```python
from build123d import *

# Parameters (mm, degrees)
F0_R     = 8.5
F1_DEPTH = 4
F2_R     = 5
F3_DEPTH = 100
F4_W     = 4
F4_H     = 5
F8_R     = 1.5
F9_DEPTH = 109.1


with BuildPart() as f1:
    # F0 (on Top) → F1 (new body)
    with BuildSketch(Plane.XY):
        Circle(F0_R)
    extrude(amount=F1_DEPTH)

    # F2 (on Top) → F3 (join)
    with BuildSketch(Plane.XY):
        Circle(F2_R)
    extrude(amount=F3_DEPTH)

    # F4 (on Right) → F5 (revolve)
    with BuildSketch(Plane.YZ):
        with Locations((2, 102.5)):
            Rectangle(F4_W, F4_H)
    revolve(axis=Axis((0, 0, 102.5), (0, 0, -1)))

    # F6 (on Right) → F7 (revolve)
    with BuildSketch(Plane.YZ):
        with BuildLine():
            ThreePointArc((3, 105), (2.12132, 107.12132), (0, 108))
            Line((0, 108), (0, 105))
            Line((0, 105), (3, 105))
        make_face()
    revolve(axis=Axis((0, 0, 106.5), (0, 0, -1)))

    # F8 (on Top) → F9 (cut)
    with BuildSketch(Plane.XY):
        Circle(F8_R)
    extrude(amount=F9_DEPTH, mode=Mode.SUBTRACT)


solid = f1.part
```
Read the model definition and answer for the solid it produces. Units are mm, in the model's axes. A direction names the side the tool comes from. Coordinates: 2 decimals unless noted, no trailing zeros. Loops run counter-clockwise (first coordinate to the right, second up) from the corner with the lowest first, then second, coordinate; pieces in that order, holes last. Notation, with made-up numbers: (70, 69.25) - (82, 69.25) arc R12 ccw to (82, 89.25) - close; hole circle Ø3 at (34.5, 53). An arc over 180 degrees is marked (long way). Answer in a Markdown table with one row per item.
1. Find section C-C, the plane x = 6. Write down the section's boundary in (y, z), then the cut area to 3 significant figures.
Conclusion:
| item | result |
|---|---|
| outline | (-6.02, 0) - (6.02, 0) - (6.02, 4) - (-6.02, 4) - close |
| area | 48.2 mm² |
2. Straight lines are drawn through the part: line 1 (Y direction, x = 0, z = 45.5); line 2 (X direction, y = 4, z = 94.5). For each, find the intervals that lie inside material, in ascending order.
Conclusion:
| item | result |
|---|---|
| line 1 | y = -5 to -1.5, 1.5 to 5 |
| line 2 | x = -3 to 3 |
3. Given pin 1 (1.5 mm diameter, centred on x = -4.5, z = 54, fed in from +Y); pin 2 (5 mm diameter, centred on x = 1, z = 90, fed in from +Y); pin 3 (2 mm diameter, centred on y = -1.5, z = 89.5, fed in from -X), each flat-ended and moving along its own axis, determine where each tip first touches the part or whether it passes through.
Conclusion:
| item | result |
|---|---|
| pin 1 | stops at y = 3.31 |
| pin 2 | stops at y = 5 |
| pin 3 | stops at x = -4.97 |
4. Find section A-A, the plane z = 45. Write down the section's boundary in (x, y).
Conclusion:
| item | result |
|---|---|
| outline | circle Ø10 at (0, 0); hole circle Ø3 at (0, 0) |
5. Determine the mould class of faces 1 (the face through (-3.905, -0.867, 102.535)), 2 (the face through (3, -1, 105)), 3 (the face through (-1.5, 0.07, 53.05)) for opening direction X: +X half, -X half, draft (parallel to the pull), parting line (faces both ways), or undercut.
Conclusion:
| item | result |
|---|---|
| face 1 | parting line |
| face 2 | draft |
| face 3 | undercut |
6. Find section B-B, the plane y = 7.25. Write down the section's boundary in (x, z).
Conclusion:
| item | result |
|---|---|
| outline | (-4.44, 0) - (4.44, 0) - (4.44, 4) - (-4.44, 4) - close |
7. Which of the six approach directions +Z, -Z, +X, -X, +Y, -Y give full straight-line access (tool end or side, diameter ignored) to faces 4 (the face through (4.57, 7.167, 1.972)), 5 (the face through (4, -4, 4))?
Conclusion:
| item | result |
|---|---|
| face 4 | +Z, -Z |
| face 5 | +Z |
